Part model, mm, in its own coordinate system. Face numbers are marked on the shaded views. A direction names the side the tool comes from. Round coordinates to 2 decimals unless told otherwise and drop trailing zeros. Order: outer loops, then holes, each group sorted by start corner. A loop starts at its lowest first (then second) coordinate and runs counter-clockwise, first axis right, second up. Notation, with made-up numbers: M 78.5,-2 L 99.5,-2 A25 cw 99.5,20 Z; hole C -21,41.5 d11. An arc over 180 degrees is marked long. One line per question, with ' | ' between items.
from build123d import *
from OCP.BRepAlgoAPI import BRepAlgoAPI_Cut
from OCP.TopTools import TopTools_ListOfShape

# Parameters (mm, degrees)
SALIENTE_EXTRUIR1_DEPTH = 5
SALIENTE_EXTRUIR2_DEPTH = 5
SALIENTE_EXTRUIR3_DEPTH = 150
CORTAR_EXTRUIR1_REACH   = 655.84
CORTAR_EXTRUIR2_REACH   = 499.984
CORTAR_EXTRUIR3_REACH   = 538.214
CROQUIS6_W              = 4.999913194
CROQUIS6_H              = 150
CORTAR_EXTRUIR4_DEPTH   = 150
CROQUIS8_R              = 5
CORTAR_EXTRUIR5_DEPTH   = 5


with BuildPart() as part:
    # Croquis1 → Saliente-Extruir1 (new body)
    with BuildSketch(Plane(origin=(0, 0, 0), x_dir=(1, 0, 0), z_dir=(0, 1, 0))):
        with BuildLine():
            Line((0, 0), (600, 0))
            ThreePointArc((600, 0), (300, 300), (0, 0))
        make_face()
    extrude(amount=-SALIENTE_EXTRUIR1_DEPTH)

    # Croquis2 → Saliente-Extruir2 (add)
    with BuildSketch(Plane.XY):
        Polygon((300, 150), (600, 0), (600, -5), (0, -5), (0, 0), align=None)
    extrude(amount=SALIENTE_EXTRUIR2_DEPTH)

    # Croquis3 → Saliente-Extruir3 (add)
    with BuildSketch(Plane(origin=(0, 0, 0), x_dir=(1, 0, 0), z_dir=(0, 1, 0))):
        Polygon((89.643082947, 213.892420268), (87.767304207, 212.03132513), (86.007761026, 210.255372485), (296.263133511, 0), (300, 0), (303.535503215, 0), (300, 3.535503215), align=None)
        Polygon((510.356917053, 213.892420268), (300, 3.535503215), (303.535503215, 0), (513.892420268, 210.356917053), (512.132034356, 212.132034356), align=None)
    extrude(amount=SALIENTE_EXTRUIR3_DEPTH)

    # Croquis4 → Cortar-Extruir1 (cut, up to next)
    with BuildSketch(Plane(origin=(148.232248392, 0, 148.232248392), x_dir=(-0.7071067811865465, 0, 0.7071067811865487), z_dir=(-0.7071067811865487, 0, -0.7071067811865465)), mode=Mode.PRIVATE) as cortar_extruir1_sk1:
        Polygon((-214.632012654, 150), (-512.121617689, 0), (-512.121617689, 150), align=None)
    cortar_extruir1_tool1 = extrude(cortar_extruir1_sk1.sketch, amount=-CORTAR_EXTRUIR1_REACH, mode=Mode.PRIVATE) & part.part
    add(cortar_extruir1_tool1.solids().sort_by_distance((440.237945, 100, -143.773448))[0], mode=Mode.SUBTRACT)

    # Croquis5 → Cortar-Extruir2 (cut, up to next)
    with BuildSketch(Plane(origin=(151.767751608, 0, -151.767751608), x_dir=(-0.7071067811865488, 0, -0.7071067811865464), z_dir=(0.7071067811865464, 0, -0.7071067811865488)), mode=Mode.PRIVATE) as cortar_extruir2_sk1:
        Polygon((-209.632056057, 150), (87.857548977, 0), (87.857548977, 150), align=None)
    cortar_extruir2_tool1 = extrude(cortar_extruir2_sk1.sketch, amount=-CORTAR_EXTRUIR2_REACH, mode=Mode.PRIVATE) & part.part
    add(cortar_extruir2_tool1.solids().sort_by_distance((159.762055, 100, -143.773448))[0], mode=Mode.SUBTRACT)

    # Croquis6 → Cortar-Extruir3 (cut, up to next)
    with BuildSketch(Plane(origin=(359.994486555, 0, -363.007018979), x_dir=(-0.7100469213351532, 0, -0.7041543648252638), z_dir=(0.7041543648252638, 0, -0.7100469213351532)), mode=Mode.PRIVATE) as cortar_extruir3_sk1:
        with Locations((-214.264032998, 75)):
            Rectangle(CROQUIS6_W, CROQUIS6_H)
    cortar_extruir3_tool1 = extrude(cortar_extruir3_sk1.sketch, amount=-CORTAR_EXTRUIR3_REACH, mode=Mode.PRIVATE) & part.part
    add(cortar_extruir3_tool1.solids().sort_by_distance((512.132004, 75, -212.132065))[0], mode=Mode.SUBTRACT)


with BuildPart() as cortar_extruir4_tool:
    # Cortar-Extruir4: read off the stored shape, not the designer's step
    # Cortar-Extruir4 outline → Cortar-Extruir4 (new body)
    with BuildSketch(Plane(origin=(0, 0, 0), x_dir=(1, 0, 0), z_dir=(0, 1, 0))):
        Polygon((87.767304207, 212.03132513), (86.192818289, 210.442155589), (89.643082947, 213.892420268), align=None)
    extrude(amount=CORTAR_EXTRUIR4_DEPTH)


with BuildPart() as part_1:
    add(part.part)

    # Cortar-Extruir4: cut by cortar_extruir4_tool, with a tolerance
    cortar_extruir4_stock = TopTools_ListOfShape()
    cortar_extruir4_stock.Append(part_1.part.wrapped)
    cortar_extruir4_tools = TopTools_ListOfShape()
    cortar_extruir4_tools.Append(cortar_extruir4_tool.part.wrapped)
    cortar_extruir4_cut = BRepAlgoAPI_Cut()
    cortar_extruir4_cut.SetArguments(cortar_extruir4_stock)
    cortar_extruir4_cut.SetTools(cortar_extruir4_tools)
    cortar_extruir4_cut.SetFuzzyValue(0.00001)
    cortar_extruir4_cut.Build()
    add(Compound.cast(cortar_extruir4_cut.Shape()).solids(), mode=Mode.REPLACE)

    # Croquis8 → Cortar-Extruir5 (cut)
    with BuildSketch(Plane.XZ.offset(5)):
        with Locations(Location((300, -15, 0), (0, 0, 270))):
            Circle(CROQUIS8_R)
    extrude(amount=-CORTAR_EXTRUIR5_DEPTH, mode=Mode.SUBTRACT)


solid = part_1.part
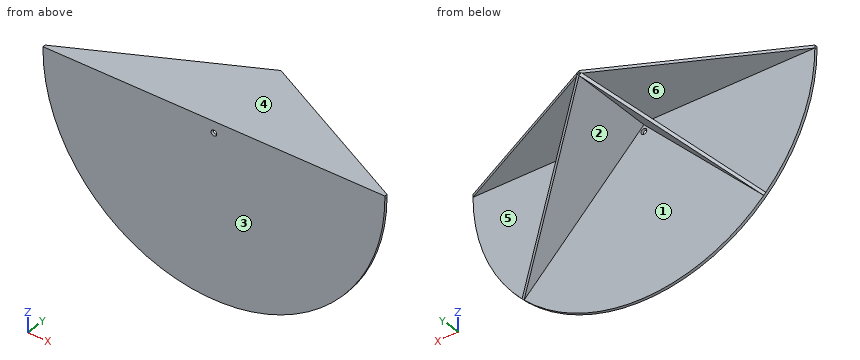
1) Probe line 1 (Z direction, x = 300, y = -2.3); line 2 (X direction, y = 76.5, z = -25); line 3 (Y direction, x = 397.5, z = -204.5). List the from-to ranges inside material, lowest first. Write a range as [from, to].
The answers:
line 1: z = [-300, -20], [-10, 5] | line 2: x = [271.26, 278.54], [321.46, 328.54] | line 3: y = [-5, 0]
2) Saw through at A-A (x = 128.5). List the corners of the cut face in (y, z).
The answers:
outline: M -5,-246.15 L 0,-246.15 L 0,-175.04 L 27.71,-175.04 L 30.3,-167.76 L 0,-167.76 L 0,0 L 64.25,0 L 64.25,5 L -5,5 Z
3) Saw through at D-D (x = 477). List the corners of the cut face in (y, z), plus the area to 3 significant figures.
The answers:
outline: M -5,-242.22 L 0,-242.22 L 0,-180.54 L 23.79,-180.54 L 26.31,-173.46 L 0,-173.46 L 0,0 L 61.5,0 L 61.5,5 L -5,5 Z | area: 1,720 mm²
4) Which spindle directions (+Z, -Z, +X, -X, +Y, -Y) get a long thin tool onto all of the face, cutting with end or side? Do the marked faces 4, 5 and 6. Say none if no direction does.
The answers:
face 4: +Z, +X, -X, +Y, -Y | face 5: +X, +Y | face 6: -X, +Y
5) Saw through at B-B (z = -103). List the corners of the cut face in (x, y), plus the area to 3 significant figures.
The answers:
outline: M 18.24,-5 L 581.76,-5 L 581.76,0 L 406.54,0 L 406.54,76.55 L 399.46,79.07 L 399.46,0 L 200.54,0 L 200.54,79.07 L 193.26,76.48 L 193.26,0 L 18.24,0 Z | area: 3,930 mm²
6) Two-plate mould, pull along X, no slides. Class the marked faces 1, 2 and 3: released by +X, released by -X, zero draft, split by the parting line, or undercut.
The answers:
face 1: undercut | face 2: undercut | face 3: zero draft
7) Saw through at C-C (y = 6). List the corners of the cut face in (x, z), plus the area to 3 significant figures.
The answers:
outline: M 12,0 L 296.26,0 L 94.42,-201.84 L 98.06,-205.48 L 300,-3.54 L 501.94,-205.48 L 505.48,-201.94 L 303.54,0 L 588,0 L 588,5 L 12,5 Z | area: 5,790 mm²
8) Drop flat-ended pins along their axis: pin 1 (12 mm diameter, centred on x = 175.5, z = -195.5, fed in from +Y); pin 2 (3 mm diameter, centred on x = 512.5, z = -212, fed in from +Y); pin 3 (1 mm diameter, centred on x = 77.5, y = 15.5, fed in from -Z). Give the stop position or say it passes through.
The answers:
pin 1: stops at y = 0 | pin 2: stops at y = 0.67 | pin 3: stops at z = 0
